Work out the finished part from the listing and answer in its coordinate system (mm). Face numbers are marked on the shaded views. Give positions to 0.01 mm unless a question says otherwise; leave off trailing zeros. Write each loop counter-clockwise with the first axis right and the second up, starting at its lowest first coordinate (ties: lowest second). Pieces come first, ordered by that corner, then holes. Notation, with made-up numbers: (73, -2.5) -> (83, -2.5) arc R17 cw to (83, 1.5) -> close; hole circle Ø2 at (62.5, 81). An arc over 180 degrees is marked (long way). Use a Markdown table: item, result. Add a question column.
Q1. Each of these flat-tipped pins is pushed along its axis until it touches: pin 1 Ø5 at (x, z) = (2, 18.5) entering from -Y; pin 2 Ø6 at (x, z) = (-3.5, 30.5) entering from +Y; pin 3 Ø8 at (x, z) = (17.5, 22) entering from -Y; pin 4 Ø1.5 at (y, z) = (-30, 42) entering from +X. Where does it stop, or does it pass through?
Q2. Section C-C, the plane z = 37 is taken. Give the vertices of the cut face in (x, y).
Q3. Section B-B, the plane x = -3.5 is taken. Give the vertices of the cut face in (y, z), plus the area to 3 significant figures.
Q4. Section D-D, the plane x = -21 is taken. Give the vertices of the cut face in (y, z), plus the area to 3 significant figures.
Q5. For a pull along X with two mould halves and no side action, classify the marked faces 1, 2 and 3 as pulls with the +X half, pulls with the -X half, needs draft (parallel to the pull), parting line crosses it, or undercut.
Q6. Section A-A, the plane y = -38 is taken. Give the vertices of the cut face in (x, z).
Q7. Consider line 1 (Y direction, x = 0, z = 48.5); line 2 (Z direction, x = -14, y = -39); line 3 (X direction, y = 23, z = 66). Determine where each line is inside the solid, lowest interval first.
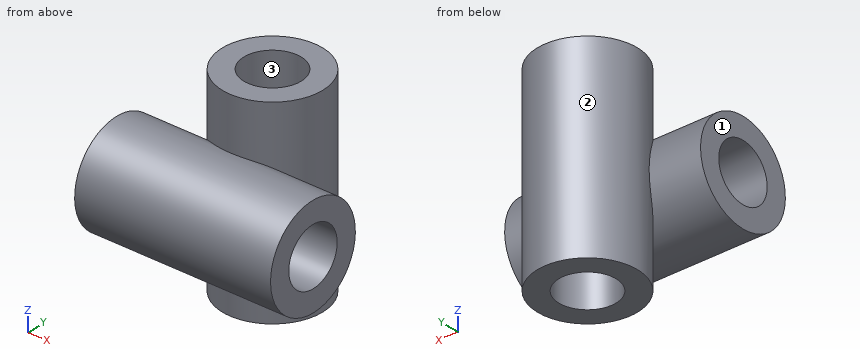
from build123d import *

# Parameters (mm, degrees)
SKETCH1_R           = 28
BOSS_EXTRUDE1_DEPTH = 110
SKETCH3_R           = 28
BOSS_EXTRUDE2_DEPTH = 55
SKETCH4_R           = 16
CUT_EXTRUDE1_DEPTH  = 140.57435311
SKETCH6_R           = 16
CUT_EXTRUDE2_DEPTH  = 169.985206622


with BuildPart() as part:
    # Sketch1 → Boss-Extrude1 (new body)
    with BuildSketch(Plane.XY):
        Circle(SKETCH1_R)
    extrude(amount=BOSS_EXTRUDE1_DEPTH)

    # Sketch3 → Boss-Extrude2 (add, symmetric)
    with BuildSketch(Plane(origin=(0, 0, 0), x_dir=(0, 0, -1), z_dir=(1, 0, 0))):
        with Locations((-54.831273686, -38)):
            Circle(SKETCH3_R)
    extrude(amount=BOSS_EXTRUDE2_DEPTH, both=True)

    # Sketch4 → Cut-Extrude1 (cut, through all)
    with BuildSketch(Plane.XY.offset(110)):
        Circle(SKETCH4_R)
    extrude(amount=-CUT_EXTRUDE1_DEPTH, mode=Mode.SUBTRACT)

    # Sketch6 → Cut-Extrude2 (cut, through all)
    with BuildSketch(Plane(origin=(55, 0, 0), x_dir=(0, 0, -1), z_dir=(1, 0, 0))):
        with Locations((-54.831273686, -38)):
            Circle(SKETCH6_R)
    extrude(amount=-CUT_EXTRUDE2_DEPTH, mode=Mode.SUBTRACT)


solid = part.part
Result set:
| question | item | result |
|---|---|---|
| 1 | pin 1 | stops at y = -28 |
| 1 | pin 2 | stops at y = 28 |
| 1 | pin 3 | stops at y = -24.53 |
| 1 | pin 4 | passes through |
| 2 | outline | (-55, -59.59) -> (55, -59.59) -> (55, -16.41) -> (22.69, -16.41) arc R28 ccw (long way) to (-22.69, -16.41) -> (-55, -16.41) -> close; hole circle Ø32 at (0, 0) |
| 3 | outline | (-27.78, 0) -> (-15.61, 0) -> (-15.61, 110) -> (-27.78, 110) -> (-27.78, 80.9) arc R28 ccw (long way) to (-27.78, 28.76) -> close; (15.61, 0) -> (27.78, 0) -> (27.78, 110) -> (15.61, 110) -> close; hole circle Ø32 at (-38, 54.83) |
| 3 | area | 3,660 mm2 |
| 4 | outline | (-18.52, 0) -> (18.52, 0) -> (18.52, 110) -> (-18.52, 110) -> (-18.52, 74.94) arc R28 ccw (long way) to (-18.52, 34.72) -> close; hole circle Ø32 at (-38, 54.83) |
| 4 | area | 5,500 mm2 |
| 5 | face 1 | pulls with the -X half |
| 5 | face 2 | parting line crosses it |
| 5 | face 3 | undercut |
| 6 | outline | (-55, 26.83) -> (55, 26.83) -> (55, 38.83) -> (-55, 38.83) -> close; (-55, 70.83) -> (55, 70.83) -> (55, 82.83) -> (-55, 82.83) -> close |
| 7 | line 1 | y = -65.27 to -52.69, -23.31 to -16, 16 to 28 |
| 7 | line 2 | z = 26.85 to 38.86, 70.8 to 82.81 |
| 7 | line 3 | x = -15.97 to 15.97 |
